Check sheet for the drawn part. Datum: minimum x, y, z corner. Units: mm. A direction names the side the tool comes from. Round coordinates to 2 decimals unless told otherwise and drop trailing zeros. Order: outer loops, then holes, each group sorted by start corner. A loop starts at its lowest first (then second) coordinate and runs counter-clockwise, first axis right, second up.
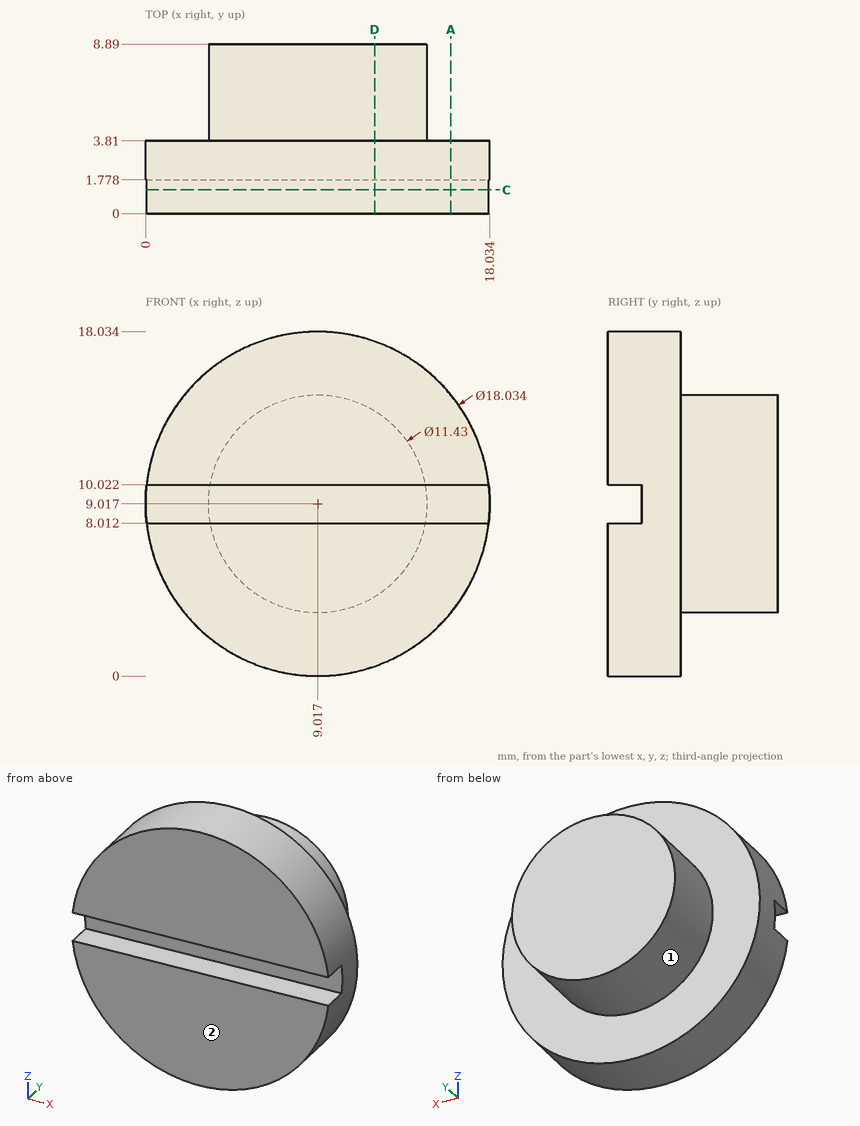
(1) Sectioned sample at A-A, the plane x = 16. Record the cut outline in (y, z), and give its area (3 significant figures).
Returned:
outline: (0, 3.31) - (3.81, 3.31) - (3.81, 14.72) - (0, 14.72) - (0, 10.02) - (1.78, 10.02) - (1.78, 8.01) - (0, 8.01) - close
area: 39.9 mm2
(2) Material ranges on line 1 (Y direction, x = 15.25, z = 5); line 2 (Z direction, x = 15.25, y = 1); line 3 (Z direction, x = 15.75, y = 1) (1 decimal), recorded low to high.
Returned:
line 1: y = 0 to 3.81
line 2: z = 2.5 to 8.01, 10.02 to 15.53
line 3: z = 3 to 8, 10 to 15
(3) Depth check by flat-ended pin: P1, Ø2, axis at y = 4, z = 2, coming from the -X side; P2, Ø0.6, axis at x = 11.5, z = 9.5, coming from the -Y side; P3, Ø0.5, axis at x = 11, y = 0.5, coming from the +Z side. Enter the tip coordinate at first touch or a pass-through.
Returned:
P1: stops at x = 2.32
P2: stops at y = 1.78
P3: stops at z = 17.87
(4) Set-up check for the marked faces 1 and 2: record each of +Z, -Z, +X, -X, +Y, -Y from which the full face is reachable in a straight line by a thin tool's end or side.
Returned:
face 1: +Y
face 2: +Z, -Z, +X, -X, -Y
(5) Sectioned sample at D-D, the plane x = 12. Record the cut outline in (y, z), and give its area (3 significant figures).
Returned:
outline: (0, 0.51) - (3.81, 0.51) - (3.81, 4.14) - (8.89, 4.14) - (8.89, 13.89) - (3.81, 13.89) - (3.81, 17.53) - (0, 17.53) - (0, 10.02) - (1.78, 10.02) - (1.78, 8.01) - (0, 8.01) - close
area: 111 mm2
(6) Sectioned sample at C-C, the plane y = 1.25. Record the cut outline in (x, z).
Returned:
outline: (0.06, 8.01) arc R9.02 ccw to (17.98, 8.01) - close; (0.06, 10.02) - (17.98, 10.02) arc R9.02 ccw to start
